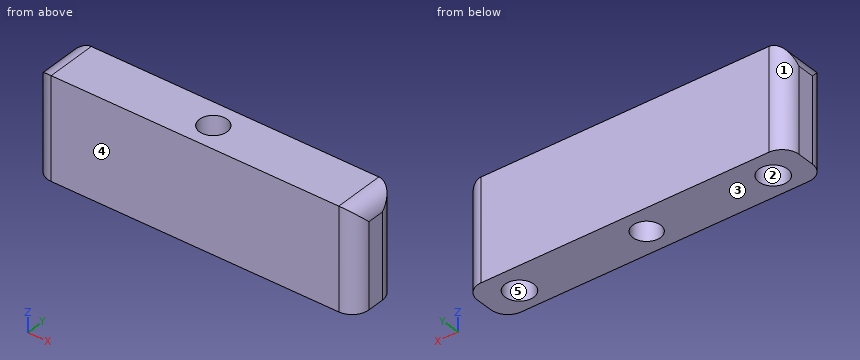
```python
from build123d import *

# Parameters (mm, degrees)
ESQUISSE1_W             = 95
ESQUISSE1_H             = 30
BOSS_EXTRU_1_DEPTH      = 15
ESQUISSE2_R             = 4.25
ENL_V_MAT_EXTRU_2_DEPTH = 20
ENL_V_MAT_EXTRU_3_REACH = 102.747
ESQUISSE3_R             = 4.1
CONG_1_R                = 5


with BuildPart() as part:
    # Esquisse1 → Boss.-Extru.1 (new body)
    with BuildSketch(Plane(origin=(0, 0, 0), x_dir=(1, 0, 0), z_dir=(0, 1, 0))):
        with Locations((-47.5, -15)):
            Rectangle(ESQUISSE1_W, ESQUISSE1_H)
    extrude(amount=BOSS_EXTRU_1_DEPTH)

    # Esquisse2 → Enlèv. mat.-Extru.2 (cut)
    with BuildSketch(Plane(origin=(0, 0, 0), x_dir=(-1, 0, 0), z_dir=(0, 0, -1))):
        with Locations((10, 7)):
            Circle(ESQUISSE2_R)
        with Locations((85, 7)):
            Circle(ESQUISSE2_R)
    extrude(amount=-ENL_V_MAT_EXTRU_2_DEPTH, mode=Mode.SUBTRACT)

    # Esquisse3 → Enlèv. mat.-Extru.3 (cut, up to next)
    with BuildSketch(Plane(origin=(0, 0, 0), x_dir=(-1, 0, 0), z_dir=(0, 0, -1)), mode=Mode.PRIVATE) as enl_v_mat_extru_3_sk1:
        with Locations((48, 7.5)):
            Circle(ESQUISSE3_R)
    enl_v_mat_extru_3_tool1 = extrude(enl_v_mat_extru_3_sk1.sketch, amount=-ENL_V_MAT_EXTRU_3_REACH, mode=Mode.PRIVATE) & part.part
    add(enl_v_mat_extru_3_tool1.solids().sort_by_distance((-48, 7.5, 0))[0], mode=Mode.SUBTRACT)

    # Congé1
    cong_1_edges = [part.edges().sort_by_distance(p)[0] for p in [
        (-95, 15, 15),
        (0, 15, 15),
        (-95, 0, 15),
        (0, 0, 15),
        (0, 7.5, 30),
        (-95, 7.5, 30),
    ]]
    fillet(cong_1_edges, radius=CONG_1_R)


solid = part.part
```
Verification items for the finished model (mm, model axes). Face numbers are marked on the shaded views. A direction names the side the tool comes from. Coordinates: 2 decimals unless noted, no trailing zeros. Order: outer loops, then holes, each group sorted by start corner. A loop starts at its lowest first (then second) coordinate and runs counter-clockwise, first axis right, second up. Notation, with made-up numbers: (13, 7.5) -> (63, 7.5) arc R15 ccw to (63, 24.5) -> close; hole circle Ø2 at (71, 37). An arc over 180 degrees is marked (long way). Put each result on its own line as item: value. Start each with the question number.
1) Go/stop test with a flat-tipped pin: pin 1 (4 mm diameter, centred on x = -83.5, y = 6, fed in from -Z). Record where the tip stops, or that it passes through.
2) Cross-section at D-D (x = -10). Enter the section's corners in (y, z).
3) Tool access check on the marked faces 1 and 2. Record the directions out of +Z, -Z, +X, -X, +Y, -Y that give a thin tool (end or side, any length) a straight path to the whole face; none if there is none.
4) Cross-section at A-A (z = 8). Enter the section's corners in (x, y).
5) Release check for a two-part mould opening along Y. For the marked faces 3, 4 and 5 record: pulls with the +Y half, pulls with the -Y half, needs draft (parallel to the pull), parting line crosses it, or undercut.
6) Cross-section at B-B (x = -48). Enter the section's corners in (y, z).
7) Cross-section at C-C (y = 9). Enter the section's corners in (x, z), plus the area to 3 significant figures.
8) Material ranges on L1, parallel to Y at x = -85, z = 7.25; L2, parallel to X at y = 6.75, z = 7; L3, parallel to Y at x = -48, z = 22, recorded low to high.
Geometry check:
1. pin 1: stops at z = 20
2. outline: (0, 0) -> (2.75, 0) -> (2.75, 20) -> (11.25, 20) -> (11.25, 0) -> (15, 0) -> (15, 30) -> (0, 30) -> close
3. face 1: +Z, -Z, -X, +Y
3. face 2: -Z
4. outline: (-95, 5) arc R5 ccw to (-90, 0) -> (-5, 0) arc R5 ccw to (0, 5) -> (0, 10) arc R5 ccw to (-5, 15) -> (-90, 15) arc R5 ccw to (-95, 10) -> close; hole circle Ø8.5 at (-85, 7); hole circle Ø8.2 at (-48, 7.5); hole circle Ø8.5 at (-10, 7)
5. face 3: needs draft
5. face 4: pulls with the -Y half
5. face 5: undercut
6. outline: (0, 0) -> (3.4, 0) -> (3.4, 30) -> (0, 30) -> close; (11.6, 0) -> (15, 0) -> (15, 30) -> (11.6, 30) -> close
7. outline: (-95, 0) -> (-88.75, 0) -> (-88.75, 20) -> (-81.25, 20) -> (-81.25, 0) -> (-51.82, 0) -> (-51.82, 30) -> (-90, 30) arc R5 ccw to (-95, 25) -> close; (-44.18, 0) -> (-13.75, 0) -> (-13.75, 20) -> (-6.25, 20) -> (-6.25, 0) -> (0, 0) -> (0, 25) arc R5 ccw to (-5, 30) -> (-44.18, 30) -> close
7. area: 2,310 mm^2
8. L1: y = 0 to 2.75, 11.25 to 15
8. L2: x = -95 to -89.24, -80.76 to -52.03, -43.97 to -14.24, -5.76 to 0
8. L3: y = 0 to 3.4, 11.6 to 15
